Design review of the part built by this model. Coordinates are the model's own, in mm. A direction names the side the tool comes from. Give positions to 0.01 mm unless a question says otherwise; leave off trailing zeros. Loops run counter-clockwise (first coordinate to the right, second up) from the corner with the lowest first, then second, coordinate; pieces in that order, holes last.
from build123d import *

# Parameters (mm, degrees)
BOSS_EXTRUDE1_START     = -9
SKETCH1_W               = 152.45
SKETCH1_H               = 16
BOSS_EXTRUDE1_DEPTH     = 5
BOSS_EXTRUDE2_START     = -9
SKETCH2_R               = 6.5
BOSS_EXTRUDE2_DEPTH     = 5
BOSS_EXTRUDE3_START     = -9
SKETCH3_R               = 8
BOSS_EXTRUDE3_DEPTH     = 5
BOSS_EXTRUDE4_START     = -9
SKETCH4_R               = 7
BOSS_EXTRUDE4_DEPTH     = 11.5
BOSS_EXTRUDE5_START     = 2.5
SKETCH5_R               = 5.5
BOSS_EXTRUDE5_DEPTH     = 1
BOSS_EXTRUDE6_START     = -4
SKETCH6_R               = 3.5
BOSS_EXTRUDE6_DEPTH     = 1
CUT_EXTRUDE1_DEPTH      = 132.004589614
CUT_EXTRUDE1_DEPTH_BACK = 132.004589614
SKETCH7_R               = 4
CUT_EXTRUDE2_DEPTH      = 132.004589614
CUT_EXTRUDE2_DEPTH_BACK = 132.004589614
SKETCH8_R               = 1.725
CUT_EXTRUDE3_DEPTH      = 132.004589614
CUT_EXTRUDE3_DEPTH_BACK = 132.004589614
SKETCH9_W               = 22.8
SKETCH9_H               = 11.9
CUT_EXTRUDE4_DEPTH      = 132.004589614
CUT_EXTRUDE4_DEPTH_BACK = 132.004589614
SKETCH10_R              = 0.9
CUT_EXTRUDE5_START      = -9
SKETCH11_R              = 2
CUT_EXTRUDE5_DEPTH      = 4


with BuildPart() as part:
    # Sketch1 → Boss-Extrude1 (new body)
    with BuildSketch(Plane.XY.offset(BOSS_EXTRUDE1_START)):
        with Locations((46.225, 0)):
            Rectangle(SKETCH1_W, SKETCH1_H)
    extrude(amount=BOSS_EXTRUDE1_DEPTH)

    # Sketch2 → Boss-Extrude2 (add)
    with BuildSketch(Plane.XY.offset(BOSS_EXTRUDE2_START)):
        with Locations((-30, 0)):
            Circle(SKETCH2_R)
    extrude(amount=BOSS_EXTRUDE2_DEPTH)

    # Sketch3 → Boss-Extrude3 (add)
    with BuildSketch(Plane.XY.offset(BOSS_EXTRUDE3_START)):
        with Locations((122.45, 0)):
            Circle(SKETCH3_R)
    extrude(amount=BOSS_EXTRUDE3_DEPTH)

    # Sketch4 → Boss-Extrude4 (add)
    with BuildSketch(Plane.XY.offset(BOSS_EXTRUDE4_START)):
        Circle(SKETCH4_R)
    extrude(amount=BOSS_EXTRUDE4_DEPTH)

    # Sketch5 → Boss-Extrude5 (add)
    with BuildSketch(Plane.XY.offset(BOSS_EXTRUDE5_START)):
        Circle(SKETCH5_R)
    extrude(amount=BOSS_EXTRUDE5_DEPTH)

    # Sketch6 → Boss-Extrude6 (add)
    with BuildSketch(Plane.XY.offset(BOSS_EXTRUDE6_START)):
        with Locations((-30, 0)):
            Circle(SKETCH6_R)
    extrude(amount=BOSS_EXTRUDE6_DEPTH)

    # Sketch7 → Cut-Extrude1 (cut, two sides: drawn at the far end of the back side and taken through both)
    with BuildSketch(Plane.XY.offset(-CUT_EXTRUDE1_DEPTH_BACK)):
        Circle(SKETCH7_R)
    extrude(amount=CUT_EXTRUDE1_DEPTH + CUT_EXTRUDE1_DEPTH_BACK, mode=Mode.SUBTRACT)

    # Sketch8 → Cut-Extrude2 (cut, two sides: drawn at the far end of the back side and taken through both)
    with BuildSketch(Plane.XY.offset(-CUT_EXTRUDE2_DEPTH_BACK)):
        with Locations((-30, 0)):
            Circle(SKETCH8_R)
    extrude(amount=CUT_EXTRUDE2_DEPTH + CUT_EXTRUDE2_DEPTH_BACK, mode=Mode.SUBTRACT)

    # Sketch9 → Cut-Extrude3 (cut, two sides: drawn at the far end of the back side and taken through both)
    with BuildSketch(Plane.XY.offset(-CUT_EXTRUDE3_DEPTH_BACK)):
        with Locations((114.2, 0)):
            Rectangle(SKETCH9_W, SKETCH9_H)
    extrude(amount=CUT_EXTRUDE3_DEPTH + CUT_EXTRUDE3_DEPTH_BACK, mode=Mode.SUBTRACT)

    # Sketch10 → Cut-Extrude4 (cut, two sides: drawn at the far end of the back side and taken through both)
    with BuildSketch(Plane.XY.offset(-CUT_EXTRUDE4_DEPTH_BACK)):
        with Locations((100.45, 0)):
            Circle(SKETCH10_R)
        with Locations((127.95, 0)):
            Circle(SKETCH10_R)
    extrude(amount=CUT_EXTRUDE4_DEPTH + CUT_EXTRUDE4_DEPTH_BACK, mode=Mode.SUBTRACT)

    # Sketch11 → Cut-Extrude5 (cut)
    with BuildSketch(Plane.XY.offset(CUT_EXTRUDE5_START)):
        with Locations((40, 0)):
            Circle(SKETCH11_R)
        with Locations((75, 0)):
            Circle(SKETCH11_R)
    extrude(amount=CUT_EXTRUDE5_DEPTH, mode=Mode.SUBTRACT)


solid = part.part
Q1. Take a section at B-B (z = -0.5). Give the boundary of the cut face in (x, y).
Results:
outline: circle Ø14 at (0, 0); hole circle Ø8 at (0, 0)
Q2. Take a section at A-A (x = 75). Give the boundary of the cut face in (y, z).
Results:
outline: (-8, -9) - (-2, -9) - (-2, -5) - (2, -5) - (2, -9) - (8, -9) - (8, -4) - (-8, -4) - close
Q3. Insertion check: pin 1 (5 mm diameter, centred on x = 83.5, y = 2, fed in from +Z); pin 2 (1.5 mm diameter, centred on y = -1, z = -7.5, fed in from -X); pin 3 (2 mm diameter, centred on y = 5, z = 1.5, fed in from -X). Each pin has a flat end and moves straight along its axis. Give the tip position at first contact, or say it passes through.
Results:
pin 1: stops at z = -4
pin 2: stops at x = -36.5
pin 3: stops at x = -5.74
Q4. Tool access review of faces 1 (the face through (6.466, -2.681, -0.796)), 2 (the face through (114, 5.95, -7)), 3 (the face through (76.908, 0.601, -7.028)): name each direction out of +Z, -Z, +X, -X, +Y, -Y from which nothing blocks a thin tool from reaching the whole face with its end or side.
Results:
face 1: +Z
face 2: +Z, -Z
face 3: -Z
Q5. Take a section at C-C (x = 51). Give the boundary of the cut face in (y, z).
Results:
outline: (-8, -9) - (8, -9) - (8, -4) - (-8, -4) - close
Q6. Wall thickness on line 1 (X direction, y = 1, z = -6.25); line 2 (X direction, y = 0, z = -1.5); line 3 (Z direction, x = 102, y = -2.5): over which ranges is each line inside the solid? List them lowest first.
Results:
line 1: x = -36.42 to -31.41, -28.59 to -3.87, 3.87 to 38.27, 41.73 to 73.27, 76.73 to 102.8, 125.6 to 130.39
line 2: x = -7 to -4, 4 to 7
line 3: z = -9 to -4
Q7. Draft analysis for pull direction X (two halves, no side actions). For faces 4 (the face through (-4, -4, 2.5)), 5 (the face through (38, 0, -7)), 6 (the face through (-0.867, -3.905, -2.838)), 7 (the face through (130.448, -0.176, -6.535)), state which applies: pulls with the +X half, pulls with the -X half, needs draft (parallel to the pull), parting line crosses it, or undercut.
Results:
face 4: needs draft
face 5: undercut
face 6: undercut
face 7: pulls with the +X half
